Geometry: see drawing. Coordinates: mm, zero at the bounding-box minimum. A direction names the side the tool comes from. Coordinates: 2 decimals unless noted, no trailing zeros. Write each loop counter-clockwise with the first axis right and the second up, starting at its lowest first coordinate (ties: lowest second). Pieces come first, ordered by that corner, then holes. Notation, with made-up numbers: (62, -23.75) - (83, -23.75) arc R28 cw to (83, 15.25) - close; hole circle Ø3 at (89, -19). An arc over 180 degrees is marked (long way). Use a Markdown table: item, result. Add a question column.
Q1. Section query A-A (x = 5). Return the cut outline in (y, z), then the cut area to 3 significant figures.
Q2. Set-up query: the marked faces 4, 5 and 6. Return all of +Z, -Z, +X, -X, +Y, -Y with unobstructed straight access to the full face (end or side cutting, diameter ignored); none if empty.
Q3. Pin query (flat end, axial travel): P1, Ø0.5, axis at x = 10.5, z = 6, coming from the +Y side; P2, Ø1, axis at x = 10.5, y = 4.5, coming from the +Z side (3 decimals); P3, Ø2, axis at x = 6, z = 7, coming from the +Y side. Return the tip coordinate at first contact, or that it passes through.
Q4. Mould query, pull axis Z, two halves, no side actions, for the marked faces 1, 2 and 3. Classes: released by +Z, released by -Z, zero draft, split by the parting line, or undercut.
Q5. Material intervals for probe 1 along Z at (x, y) = (10.25, 7.25); probe 2 along X at (y, z) = (8.5, 5.5); probe 3 along Z at (x, y) = (3.5, 5.75), sorted ascending. Write a range as from..to.
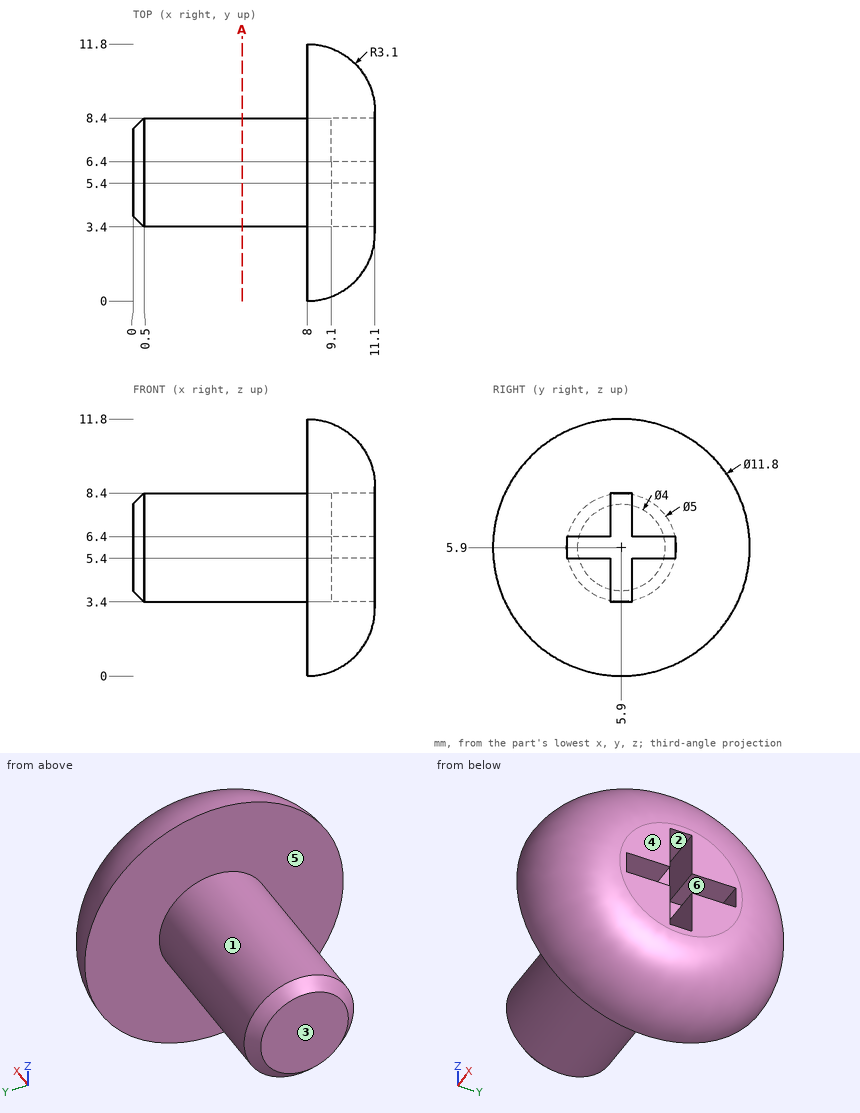
Values follow:
| question | item | result |
|---|---|---|
| 1 | outline | circle Ø5 at (5.9, 5.9) |
| 1 | area | 19.6 mm2 |
| 2 | face 4 | +Z, -Z, +X, +Y, -Y |
| 2 | face 5 | -X |
| 2 | face 6 | +X |
| 3 | P1 | y = 10.83 |
| 3 | P2 | z = 10.895 |
| 3 | P3 | y = 8.4 |
| 4 | face 1 | split by the parting line |
| 4 | face 2 | undercut |
| 4 | face 3 | zero draft |
| 5 | probe 1 | 1.16..5.4, 6.4..10.64 |
| 5 | probe 2 | 8..11.1 |
| 5 | probe 3 | 3.4..8.4 |
